Could you check a few things on this model? Use its own coordinates, in mm. A direction names the side the tool comes from. Coordinates: 2 decimals unless noted, no trailing zeros. Write each loop counter-clockwise with the first axis right and the second up, starting at its lowest first coordinate (ties: lowest second). Pieces come first, ordered by that corner, then holes. Notation, with made-up numbers: M -32,43.5 L -25,43.5 A20 ccw -25,62.5 Z; hole C 82.5,-30.5 d10. An arc over 180 degrees is marked long. Answer as CSV lines item,"result". Start each with the question number.
Item 1: We'd pull the mould along Z, two halves only. Please class faces 1 (the cylindrical face through (-53.096, 2.958, -39.96)), 2 (the flat face through (-60.429, 3, -34)), 3 (the flat face through (68, 3, -28.598)): +Z half, -Z half, draft (parallel to the pull), parting line (faces both ways), or undercut.
Item 2: If I drill on line 1 along X through (y, z) = (1.2, -9); line 2 along Z through (x, y) = (-49.5, 3.65); line 3 along X through (y, z) = (4.15, -6), over which ranges is the centre line in solid material (lowest first)? Write a range as [from, to].
Item 3: I'm going to push flat-ended pins straight in: P1, Ø3, axis at x = 68, y = 2.5, coming from the +Z side; P2, Ø1.8, axis at x = -32.5, y = 3.5, coming from the +Z side; P3, Ø3, axis at y = 2, z = -5.5, coming from the +X side; P4, Ø2, axis at x = 36, z = -26.5, coming from the -Y side. Where does each tip first touch, or does it pass through?
Item 4: Suppose I cut it at A-A, the plane y = 4.05. Write out the boundary of the cut face in (x, z), and give its area (3 significant figures).
Item 5: On a 3-axis mill with a long thin cutter (end or side, diameter ignored), from which of +Z, -Z, +X, -X, +Y, -Y can I reach the whole of each face in a straight line? I mean faces 4 (the flat face through (19.738, 3, -6)), 5 (the flat face through (-54.429, 3, -17)), 6 (the flat face through (68, 3, -38.598)). Say none if no direction works.
Item 6: Suppose I cut it at C-C, the plane z = -20.5. Write out the boundary of the cut face in (x, y), and give its area (3 significant figures).
Item 7: Suppose I cut it at B-B, the plane x = 50.5. Write out the boundary of the cut face in (y, z), and give its area (3 significant figures).
Autodesk Inventor part; units mm, degrees
ref_plane "YZ Plane" through (0, 0, 0) normal (1, 0, 0) x (0, 1, 0)
ref_plane "XZ Plane" through (0, 0, 0) normal (0, 1, 0) x (-1, 0, 0)
ref_plane "XY Plane" through (0, 0, 0) normal (0, 0, 1) x (1, 0, 0)
sketch "Sketch1" plane through (0, 0, 0) normal (0, 1, 0) x (-1, 0, 0)
  line L0 (54.4292, -43.2642) -> (54.4292, -41.2642)
  arc A0 (54.4292, -38.5976) -> (54.4292, -41.2642) centre (54.4292, -39.9309) ccw
  arc A1 (54.4292, -25.9309) -> (54.4292, -28.5976) centre (54.4292, -27.2642) ccw
  line L1 (54.4292, -25.9309) -> (54.4292, -8.5976)
  line L2 (54.4292, -28.5976) -> (60.4292, -28.5976)
  line L3 (54.4292, -38.5976) -> (60.4292, -38.5976)
  line L4 (60.4292, -38.5976) -> (60.4292, -28.5976)
  line L5 (54.4292, -43.2642) -> (-65.0708, -43.2642)
  line L6 (-65.0708, -43.2642) -> (-65.0708, -41.2642)
  arc A2 (-65.0708, -41.2642) -> (-65.0708, -38.5976) centre (-65.0708, -39.9309) ccw
  arc A3 (-65.0708, -28.5976) -> (-65.0708, -25.9309) centre (-65.0708, -27.2642) ccw
  line L7 (-65.0708, -25.9309) -> (-65.0708, -8.5976)
  line L8 (-65.0708, -28.5976) -> (-71.0708, -28.5976)
  line L9 (-65.0708, -38.5976) -> (-71.0708, -38.5976)
  line L10 (-71.0708, -38.5976) -> (-71.0708, -28.5976)
  arc A4 (9.0959, -8.5976) -> (10.4292, -8.5976) centre (9.7625, -8.5976) ccw
  arc A5 (-21.0708, -8.5976) -> (-19.7375, -8.5976) centre (-20.4041, -8.5976) ccw
  line L11 (-21.0708, -8.5976) -> (-65.0708, -8.5976)
  line L12 (54.4292, -8.5976) -> (10.4292, -8.5976)
  line L13 (-19.7375, -2.5976) -> (9.0959, -2.5976)
  line L14 (-19.7375, -8.5976) -> (-19.7375, -2.5976)
  line L15 (9.0959, -8.5976) -> (9.0959, -2.5976)
  point P0 (0, 0)
  dimension "d1" = 2
  dimension "d2" = 2.6667
  dimension "d5" = 2.6667
  dimension "d6" = 17.3333
  dimension "d9" = 6
  dimension "d10" = 119.5
  dimension "d11" = 10
  dimension "d15" = 1.3333
  dimension "d16" = 1.3333
  dimension "d18" = 44
  dimension "d19" = 44
  dimension "d21" = 20
  dimension "d23" = 6
extrude "Extrusion1" add sketch "Sketch1" along normal blind 6
properties part number "Support A Cross" material "Wood (Maple)"
Ans:
1,face 1,"undercut"
1,face 2,"draft"
1,face 3,"+Z half"
2,line 1,"x = [-54.43, -10.29], [-9.23, 19.87], [20.94, 65.07]"
2,line 2,"z = [-43.26, -8.6]"
2,line 3,"x = [-9.1, 19.74]"
3,P1,"stops at z = -28.6"
3,P2,"stops at z = -8.6"
3,P3,"stops at x = 19.74"
3,P4,"stops at y = 0"
4,outline,"M -60.43,-38.6 L -54.43,-38.6 A1.33 cw -54.43,-41.26 L -54.43,-43.26 L 65.07,-43.26 L 65.07,-41.26 A1.33 cw 65.07,-38.6 L 71.07,-38.6 L 71.07,-28.6 L 65.07,-28.6 A1.33 cw 65.07,-25.93 L 65.07,-8.6 L 21.07,-8.6 A0.67 cw 19.74,-8.6 L 19.74,-2.6 L -9.1,-2.6 L -9.1,-8.6 A0.67 cw -10.43,-8.6 L -54.43,-8.6 L -54.43,-25.93 A1.33 cw -54.43,-28.6 L -60.43,-28.6 Z"
4,area,"4,420 mm^2"
5,face 4,"+Z, +X, +Y, -Y"
5,face 5,"+Z, -X, +Y, -Y"
5,face 6,"-Z, +X, +Y, -Y"
6,outline,"M -54.43,0 L 65.07,0 L 65.07,6 L -54.43,6 Z"
6,area,"717 mm^2"
7,outline,"M 0,-43.26 L 6,-43.26 L 6,-8.6 L 0,-8.6 Z"
7,area,"208 mm^2"
